Here's how the part is built. I have some questions about the finished solid (model axes, mm). A direction names the side the tool comes from. Round coordinates to 2 decimals unless told otherwise and drop trailing zeros. Write each loop counter-clockwise with the first axis right and the second up, starting at its lowest first coordinate (ties: lowest second). Pieces come first, ordered by that corner, then holes. Notation, with made-up numbers: (-21, -39) -> (12, -39) arc R29 ccw to (12, -10) -> close; hole circle Ø4 at (-22, -34). An arc over 180 degrees is marked (long way). Put each result on its own line as item: value. Start each with the question number.
1. Suppose I cut it at D-D (x = -17). Please give me the cut outline in (y, z).
2. Suppose I cut it at A-A (z = 0). Please give me the cut outline in (x, y), then the cut area to 3 significant figures.
3. I need wall thicknesses on probe 1 along X at (y, z) = (5.15, 15); probe 2 along X at (y, z) = (2.55, 15); probe 3 along Z at (x, y) = (-2.5, 1.5). Which ranges of each line are inside material? Lowest first, please. Write a range as from..to.
4. Suppose I cut it at C-C (y = 11.5). Please give me the cut outline in (x, z) (3 decimals).
5. Suppose I cut it at B-B (z = -30). Please give me the cut outline in (x, y).
6. For pin 1 (5.5 mm diameter, centred on x = 0, z = -30, fed in from +Y); pin 2 (3 mm diameter, centred on x = -39.5, z = 22, fed in from -Y); pin 3 (2.5 mm diameter, centred on x = -38.11, z = 22, fed in from -Y); pin 4 (8 mm diameter, centred on x = -0.5, y = 2, fed in from +Z), each with a flat end and sliding along its axis, tell me the tip position at first contact or that it passes through.
7. Which directions (+Z, -Z, +X, -X, +Y, -Y) give clear straight access to the entire face, cutting with the end or side of a thin tool? Please do faces 1 (the face through (-2.39, 1.28, -45.36)), 2 (the face through (1, 7.5, -4)), 3 (the face through (-20, 5, 31)), 4 (the face through (41.07, 7.89, 16.72)).
8. We'd pull the mould along Z, two halves only. Please class faces 5 (the face through (0, 4, 24.495)), 6 (the face through (-20.6, 0.57, 30.63)), 7 (the face through (28.932, 1.972, 13.118)): +Z half, -Z half, draft (parallel to the pull), parting line (faces both ways), or undercut.
```python
from build123d import *

# Parameters (mm, degrees)
SKETCH_1_R          = 40
EXTRUDE_1_DEPTH     = 16
SKETCH_2_R          = 37
CUT_EXTRUDE_1_DEPTH = 8.5
SKETCH_3_W          = 40
SKETCH_3_H          = 14.857277492
CUT_EXTRUDE_2_DEPTH = 59.787753827
SKETCH_4_W          = 40
SKETCH_4_H          = 3
CUT_EXTRUDE_3_DEPTH = 59.787753827
SKETCH_5_R          = 1.75
CUT_EXTRUDE_4_DEPTH = 59.787753827
EXTRUDE_2_DEPTH     = 16
SKETCH_10_R         = 1.45
CUT_EXTRUDE_5_DEPTH = 68.772200298
CUT_EXTRUDE_6_DEPTH = 2.6
SKETCH_13_R         = 3.5
CUT_EXTRUDE_7_DEPTH = 4
FILLET_2_R          = 2
FILLET_3_R          = 2


with BuildPart() as part:
    # 草图1 → 凸台-拉伸1 (new body)
    with BuildSketch(Plane(origin=(0, 0, 0), x_dir=(1, 0, 0), z_dir=(0, 1, 0))):
        with Locations(Location((0, 0, 0), (0, 0, 270))):
            Circle(SKETCH_1_R)
    extrude(amount=EXTRUDE_1_DEPTH)

    # 草图2 → 切除-拉伸1 (cut)
    with BuildSketch(Plane(origin=(0, 16, 0), x_dir=(1, 0, 0), z_dir=(0, 1, 0))):
        with Locations(Location((0, 0, 0), (0, 0, 270))):
            Circle(SKETCH_2_R)
    extrude(amount=-CUT_EXTRUDE_1_DEPTH, mode=Mode.SUBTRACT)

    # 草图3 → 切除-拉伸2 (cut, through all)
    with BuildSketch(Plane.XZ):
        with Locations((0, 34.924092916)):
            Rectangle(SKETCH_3_W, SKETCH_3_H)
    extrude(amount=-CUT_EXTRUDE_2_DEPTH, mode=Mode.SUBTRACT)

    # 草图4 → 切除-拉伸3 (cut, through all)
    with BuildSketch(Plane.XZ):
        with Locations((0, 25.99545417)):
            Rectangle(SKETCH_4_W, SKETCH_4_H)
    extrude(amount=-CUT_EXTRUDE_3_DEPTH, mode=Mode.SUBTRACT)

    # 草图5 → 切除-拉伸4 (cut, through all)
    with BuildSketch(Plane.XZ):
        with Locations(Location((0, -30, 0), (0, 0, 270))):
            Circle(SKETCH_5_R)
        with Locations(Location((-25.980762114, 15, 0), (0, 0, 270))):
            Circle(SKETCH_5_R)
        with Locations(Location((25.980762114, 15, 0), (0, 0, 270))):
            Circle(SKETCH_5_R)
    extrude(amount=-CUT_EXTRUDE_4_DEPTH, mode=Mode.SUBTRACT)

    # 草图6 → 凸台-拉伸2 (add)
    with BuildSketch(Plane.XZ):
        Polygon((29.32705693, 27.20983301), (38.222924566, 11.79016699), (43.999676996, 21.788290048), (40.874061704, 27.206080183), align=None)
        Polygon((8.900878155, -39.002892824), (-8.900878155, -38.997107176), (-3.130625811, -48.998983061), (3.124125724, -49.001015883), align=None)
        Polygon((-38.227935084, 11.793059814), (-29.322046411, 27.206940186), (-40.869051185, 27.210693013), (-43.998187428, 21.7949357), align=None)
    extrude(amount=-EXTRUDE_2_DEPTH)

    # 草图10 → 切除-拉伸5 (cut, through all)
    with BuildSketch(Plane(origin=(0, 16, 0), x_dir=(1, 0, 0), z_dir=(0, 1, 0))):
        with Locations(Location((0.000113428, 44.000000301, 0), (0, 0, 270))):
            Circle(SKETCH_10_R)
        with Locations(Location((38.105061313, -22.000098382, 0), (0, 0, 270))):
            Circle(SKETCH_10_R)
        with Locations(Location((-38.105174741, -21.999901919, 0), (0, 0, 270))):
            Circle(SKETCH_10_R)
    extrude(amount=-CUT_EXTRUDE_5_DEPTH, mode=Mode.SUBTRACT)

    # 草图11 → 切除-拉伸6 (cut)
    with BuildSketch(Plane.XZ):
        Polygon((-39.692887981, 19.249901919), (-36.517461501, 19.249901919), (-34.929748261, 21.999901919), (-36.517461501, 24.749901919), (-39.692887981, 24.749901919), (-41.280601222, 21.999901919), align=None)
        Polygon((3.175539908, -44.000000301), (1.587826668, -41.250000301), (-1.587599812, -41.250000301), (-3.175313053, -44.000000301), (-1.587599812, -46.750000301), (1.587826668, -46.750000301), align=None)
        Polygon((36.517348073, 24.750098382), (34.929634833, 22.000098382), (36.517348073, 19.250098382), (39.692774553, 19.250098382), (41.280487794, 22.000098382), (39.692774553, 24.750098382), align=None)
    extrude(amount=-CUT_EXTRUDE_6_DEPTH, mode=Mode.SUBTRACT)

    # 草图13 → 切除-拉伸7 (cut)
    with BuildSketch(Plane.XZ):
        with Locations(Location((-25.980762114, 15, 0), (0, 0, 270))):
            Circle(SKETCH_13_R)
        with Locations(Location((25.980762114, 15, 0), (0, 0, 270))):
            Circle(SKETCH_13_R)
        with Locations(Location((0, -30, 0), (0, 0, 270))):
            Circle(SKETCH_13_R)
    extrude(amount=-CUT_EXTRUDE_7_DEPTH, mode=Mode.SUBTRACT)

    # 圆角2
    fillet_2_edges = [part.edges().sort_by_distance(p)[0] for p in [
        (20, 7.5, 27.812109501),
        (-20, 7.5, 27.812109501),
        (-20, 0, 29.568235161),
        (20, 0, 29.568235161),
        (0, 7.5, 24.49545417),
        (-20, 3.75, 24.49545417),
        (20, 3.75, 24.49545417),
        (0, 0, 24.49545417),
    ]]
    fillet(fillet_2_edges, radius=FILLET_2_R)

    # 圆角3
    fillet_3_edges = [part.edges().sort_by_distance(p)[0] for p in [
        (-20, 16, 32.884890492),
        (-20, 10.75, 31.128764833),
        (20, 10.75, 31.128764833),
        (20, 16, 32.884890492),
    ]]
    fillet(fillet_3_edges, radius=FILLET_3_R)


solid = part.part
```
Verdict:
1. outline: (0, -36.21) -> (16, -36.21) -> (16, -32.86) -> (7.5, -32.86) -> (7.5, 22.5) arc R2 ccw to (5.5, 24.5) -> (2, 24.5) arc R2 ccw to (0, 22.5) -> close
2. outline: (-40, 0) -> (40, 0) -> (40, 16) -> (37, 16) -> (37, 7.5) -> (-37, 7.5) -> (-37, 16) -> (-40, 16) -> close
2. area: 651 mm^2
3. probe 1: x = -40.08..-27.73, -24.23..24.23, 27.73..40.08
3. probe 2: x = -40.08..-29.48, -22.48..22.48, 29.48..40.08
3. probe 3: z = -49..-45.17, -42.83..-32.45, -27.55..24.43
4. outline: (-43.998, 21.795) -> (-38.228, 11.793) -> (-38.215, 11.815) arc R40 ccw to (-8.901, -38.997) -> (-3.131, -48.999) -> (3.124, -49.001) -> (8.901, -39.003) -> (8.876, -39.003) arc R40 ccw to (38.223, 11.79) -> (44, 21.788) -> (40.874, 27.206) -> (29.327, 27.21) -> (29.34, 27.188) arc R40 ccw to (20, 34.641) -> (20, 32.202) arc R2 ccw to (20.872, 30.551) arc R37 cw (long way) to (-20.872, 30.551) arc R2 ccw to (-20, 32.202) -> (-20, 34.641) arc R40 ccw to (-29.322, 27.207) -> (-40.869, 27.211) -> close; hole circle Ø2.9 at (-38.105, 22); hole circle Ø2.9 at (0, -44); hole circle Ø2.9 at (38.105, 22)
5. outline: (-26.46, 0) -> (-3.5, 0) -> (-3.5, 4) -> (-1.75, 4) -> (-1.75, 7.5) -> (-21.66, 7.5) -> (-21.66, 16) -> (-26.46, 16) -> close; (1.75, 4) -> (3.5, 4) -> (3.5, 0) -> (26.46, 0) -> (26.46, 16) -> (21.66, 16) -> (21.66, 7.5) -> (1.75, 7.5) -> close
6. pin 1: stops at y = 7.5
6. pin 2: stops at y = 2.6
6. pin 3: passes through
6. pin 4: stops at z = 24.5
7. face 1: -Y
7. face 2: +Y
7. face 3: +Z, +Y, -Y
7. face 4: +X, +Y, -Y
8. face 5: +Z half
8. face 6: draft
8. face 7: undercut
